```python
from build123d import *

# Parameters (mm, degrees)
ESQUISSE1_W             = 25
ESQUISSE1_H             = 25
BOSS_EXTRU_1_DEPTH      = 95
ESQUISSE2_W             = 130
ESQUISSE2_H             = 45
BOSS_EXTRU_2_DEPTH      = 10
ESQUISSE4_W             = 10
ESQUISSE4_H             = 120
BOSS_EXTRU_3_DEPTH      = 45
ESQUISSE5_R             = 5
ENL_V_MAT_EXTRU_1_DEPTH = 235.747204456
ESQUISSE6_R             = 9.997992339
ENL_V_MAT_EXTRU_2_DEPTH = 10


with BuildPart() as part:
    # Esquisse1 → Boss.-Extru.1 (new body)
    with BuildSketch(Plane.XY):
        with Locations((-12.5, -12.5)):
            Rectangle(ESQUISSE1_W, ESQUISSE1_H)
    extrude(amount=BOSS_EXTRU_1_DEPTH)

    # Esquisse2 → Boss.-Extru.2 (add)
    with BuildSketch(Plane.XY.offset(95)):
        with Locations((-12.5, -12.5)):
            Rectangle(ESQUISSE2_W, ESQUISSE2_H)
    extrude(amount=BOSS_EXTRU_2_DEPTH)

    # Esquisse4 → Boss.-Extru.3 (add)
    with BuildSketch(Plane(origin=(0, 10, 0), x_dir=(1, 0, 0), z_dir=(0, 1, 0))):
        with Locations((-82.5, -155)):
            Rectangle(ESQUISSE4_W, ESQUISSE4_H)
        with Locations((57.5, -155)):
            Rectangle(ESQUISSE4_W, ESQUISSE4_H)
    extrude(amount=-BOSS_EXTRU_3_DEPTH)

    # Esquisse5 → Enlèv. mat.-Extru.1 (cut, through all)
    with BuildSketch(Plane(origin=(0, 0, 0), x_dir=(1, 0, 0), z_dir=(0, 1, 0))):
        with Locations(Location((-12.5, -20, 0), (0, 0, 270))):
            Circle(ESQUISSE5_R)
    extrude(amount=-ENL_V_MAT_EXTRU_1_DEPTH, mode=Mode.SUBTRACT)

    # Esquisse6 → Enlèv. mat.-Extru.2 (cut)
    with BuildSketch(Plane.XZ.offset(25)):
        with Locations(Location((-12.5, 20, 0), (0, 0, 270))):
            Circle(ESQUISSE6_R)
    extrude(amount=-ENL_V_MAT_EXTRU_2_DEPTH, mode=Mode.SUBTRACT)


solid = part.part
```
Could you check a few things on this model? Use its own coordinates, in mm. A direction names the side the tool comes from. Coordinates: 2 decimals unless noted, no trailing zeros. Write each loop counter-clockwise with the first axis right and the second up, starting at its lowest first coordinate (ties: lowest second). Pieces come first, ordered by that corner, then holes. Notation, with made-up numbers: (67, 78) - (83, 78) arc R21 cw to (83, 96) - close; hole circle Ø8 at (-4.75, 11). An arc over 180 degrees is marked (long way). Use a Markdown table: item, result.
Q1. Please list where these lines run through material, in increasing order: L1, parallel to X at y = -2, z = 113; L2, parallel to Z at x = -12, y = -23; L3, parallel to X at y = -3.5, z = 20.
Geometry check:
| item | result |
|---|---|
| L1 | x = -87.5 to -77.5, 52.5 to 62.5 |
| L2 | z = 0 to 10.01, 29.99 to 105 |
| L3 | x = -25 to -17.5, -7.5 to 0 |
Q2. I'm going to push flat-ended pins straight in: pin 1 Ø16 at (x, z) = (-12.5, 20) entering from -Y; pin 2 Ø3 at (x, y) = (45, -4.5) entering from +Z; pin 3 Ø8 at (y, z) = (-18.5, 89) entering from +X. Where does each tip first touch, or does it pass through?
Geometry check:
| item | result |
|---|---|
| pin 1 | stops at y = -15 |
| pin 2 | stops at z = 105 |
| pin 3 | stops at x = 0 |
Q3. Which directions (+Z, -Z, +X, -X, +Y, -Y) give clear straight access to the entire face, cutting with the end or side of a thin tool? Please do faces 5 (the flat face through (-77.5, -12, 161)), 6 (the flat face through (0, -13, 47)), 7 (the flat face through (-13, -25, 47)), 8 (the cylindrical face through (-16.329, -20.07, 10.764)), 9 (the flat face through (-13, 0, 47)).
Geometry check:
| item | result |
|---|---|
| face 5 | +Z, +Y, -Y |
| face 6 | -Z, +X, +Y, -Y |
| face 7 | -Z, +X, -X, -Y |
| face 8 | -Y |
| face 9 | -Z, +X, -X, +Y |
Q4. Imagine slicing it at A-A (z = 20). List the corners of the cut face in (x, y) for me.
Geometry check:
| item | result |
|---|---|
| outline | (-25, -25) - (-22.5, -25) - (-22.5, -15) - (-17.5, -15) - (-17.5, 0) - (-25, 0) - close; (-7.5, -15) - (-2.5, -15) - (-2.5, -25) - (0, -25) - (0, 0) - (-7.5, 0) - close |
Q5. Imagine slicing it at D-D (z = 148). List the corners of the cut face in (x, y) for me, and give its area (3 significant figures).
Geometry check:
| item | result |
|---|---|
| outline | (-87.5, -35) - (-77.5, -35) - (-77.5, 10) - (-87.5, 10) - close; (52.5, -35) - (62.5, -35) - (62.5, 10) - (52.5, 10) - close |
| area | 900 mm2 |
Q6. Imagine slicing it at B-B (x = -12.5). List the corners of the cut face in (y, z) for me, and give its area (3 significant figures).
Geometry check:
| item | result |
|---|---|
| outline | (-35, 95) - (-25, 95) - (-25, 30) - (-15, 30) - (-15, 25) - (0, 25) - (0, 95) - (10, 95) - (10, 105) - (-35, 105) - close; (-25, 0) - (0, 0) - (0, 15) - (-15, 15) - (-15, 10) - (-25, 10) - close |
| area | 2,480 mm2 |
Q7. Imagine slicing it at C-C (y = -6). List the corners of the cut face in (x, z) for me, and give its area (3 significant figures).
Geometry check:
| item | result |
|---|---|
| outline | (-87.5, 95) - (-25, 95) - (-25, 0) - (0, 0) - (0, 95) - (62.5, 95) - (62.5, 215) - (52.5, 215) - (52.5, 105) - (-77.5, 105) - (-77.5, 215) - (-87.5, 215) - close; hole circle Ø10 at (-12.5, 20) |
| area | 6,000 mm2 |
Q8. Thinking about a two-plate mould opening in X: for faces 1 (the flat face through (52.5, -12, 161)), 2 (the flat face through (-25, -13, 47)), 3 (the flat face through (-15, -15, 25)), 4 (the flat face through (57, -12, 215)), which applies, +X half, -X half, draft (parallel to the pull), parting line (faces both ways), or undercut?
Geometry check:
| item | result |
|---|---|
| face 1 | undercut |
| face 2 | -X half |
| face 3 | undercut |
| face 4 | draft |
